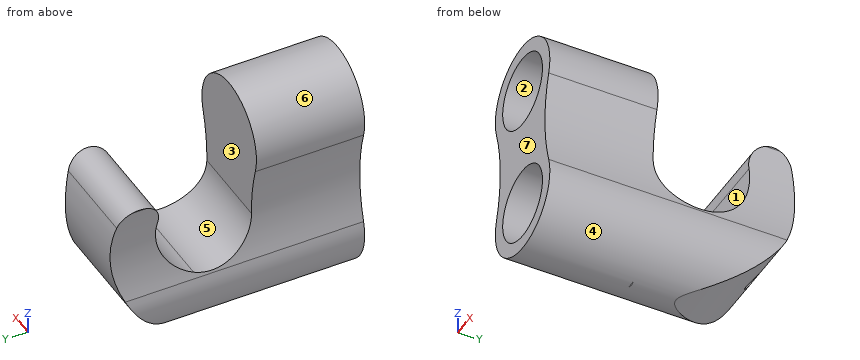
from build123d import *

# Parameters (mm, degrees)
F0_R     = 10.922
F1_DEPTH = 25.4
F2_DEPTH = 6.35
F4_DEPTH = 25.4
F5_DEPTH = 76.2
F6_DEPTH = 25.4
F7_D     = 5.4102
F8_R     = 12.7


with BuildPart() as f1:
    # F0 (on Front) → F1 (new body)
    with BuildSketch(Plane.XZ):
        with BuildLine():
            ThreePointArc((14.3656110791, 14.4652509653), (0, 3.7465), (-14.3656110791, 14.4652509653))
            ThreePointArc((-14.3656110791, 14.4652509653), (-12.2625977878, 0), (-14.3656110791, -14.4652509653))
            ThreePointArc((-14.3656110791, -14.4652509653), (0, -3.7465), (14.3656110791, -14.4652509653))
            ThreePointArc((14.3656110791, -14.4652509653), (12.2625977878, 0), (14.3656110791, 14.4652509653))
        make_face()
        with BuildLine():
            ThreePointArc((14.3656110791, 14.4652509653), (14.8300917669, 16.5764447631), (14.986, 18.7325))
            ThreePointArc((14.986, 18.7325), (-2.1560552369, 33.5625917669), (-14.3656110791, 14.4652509653))
            ThreePointArc((-14.3656110791, 14.4652509653), (0, 3.7465), (14.3656110791, 14.4652509653))
        make_face()
        with Locations((0, 18.7325)):
            Circle(F0_R, mode=Mode.SUBTRACT)
        with BuildLine():
            ThreePointArc((14.3656110791, -14.4652509653), (0, -3.7465), (-14.3656110791, -14.4652509653))
            ThreePointArc((-14.3656110791, -14.4652509653), (-2.1560552369, -33.5625917669), (14.986, -18.7325))
            ThreePointArc((14.986, -18.7325), (14.8300917669, -16.5764447631), (14.3656110791, -14.4652509653))
        make_face()
        with Locations((0, -18.7325)):
            Circle(F0_R, mode=Mode.SUBTRACT)
    extrude(amount=F1_DEPTH)

    # F0 (on Front) → F2 (join)
    with BuildSketch(Plane.XZ):
        with BuildLine():
            ThreePointArc((14.3656110791, 14.4652509653), (14.8300917669, 16.5764447631), (14.986, 18.7325))
            ThreePointArc((14.986, 18.7325), (-2.1560552369, 33.5625917669), (-14.3656110791, 14.4652509653))
            ThreePointArc((-14.3656110791, 14.4652509653), (0, 3.7465), (14.3656110791, 14.4652509653))
        make_face()
        with Locations((0, 18.7325)):
            Circle(F0_R, mode=Mode.SUBTRACT)
        with BuildLine():
            ThreePointArc((14.3656110791, 14.4652509653), (0, 3.7465), (-14.3656110791, 14.4652509653))
            ThreePointArc((-14.3656110791, 14.4652509653), (-12.2625977878, 0), (-14.3656110791, -14.4652509653))
            ThreePointArc((-14.3656110791, -14.4652509653), (0, -3.7465), (14.3656110791, -14.4652509653))
            ThreePointArc((14.3656110791, -14.4652509653), (12.2625977878, 0), (14.3656110791, 14.4652509653))
        make_face()
        with BuildLine():
            ThreePointArc((14.3656110791, -14.4652509653), (0, -3.7465), (-14.3656110791, -14.4652509653))
            ThreePointArc((-14.3656110791, -14.4652509653), (-2.1560552369, -33.5625917669), (14.986, -18.7325))
            ThreePointArc((14.986, -18.7325), (14.8300917669, -16.5764447631), (14.3656110791, -14.4652509653))
        make_face()
        with Locations((0, -18.7325)):
            Circle(F0_R, mode=Mode.SUBTRACT)
        with Locations((0, 18.7325)):
            Circle(F0_R)
        with Locations((0, -18.7325)):
            Circle(F0_R)
    extrude(amount=-F2_DEPTH)

    # F3 (on Right) → F4 (join, symmetric)
    with BuildSketch(Plane.YZ):
        with BuildLine():
            Line((0, 0), (6.35, -33.6685143411))
            ThreePointArc((6.35, -33.6685143411), (38.7816728167, -23.0090487153), (46.444249479, 10.2583907415))
            ThreePointArc((46.444249479, 10.2583907415), (38.5562501556, 14.5507638234), (34.2638770738, 6.6627644999))
            ThreePointArc((34.2638770738, 6.6627644999), (20.4633207868, -13.8005562869), (0, 0))
        make_face()
    extrude(amount=F4_DEPTH, both=True)

    # F0 (on Front) → F5 (intersect)
    with BuildSketch(Plane.XZ):
        with BuildLine():
            ThreePointArc((14.3656110791, 14.4652509653), (14.8300917669, 16.5764447631), (14.986, 18.7325))
            ThreePointArc((14.986, 18.7325), (-2.1560552369, 33.5625917669), (-14.3656110791, 14.4652509653))
            ThreePointArc((-14.3656110791, 14.4652509653), (0, 3.7465), (14.3656110791, 14.4652509653))
        make_face()
        with Locations((0, 18.7325)):
            Circle(F0_R, mode=Mode.SUBTRACT)
        with BuildLine():
            ThreePointArc((14.3656110791, 14.4652509653), (0, 3.7465), (-14.3656110791, 14.4652509653))
            ThreePointArc((-14.3656110791, 14.4652509653), (-12.2625977878, 0), (-14.3656110791, -14.4652509653))
            ThreePointArc((-14.3656110791, -14.4652509653), (0, -3.7465), (14.3656110791, -14.4652509653))
            ThreePointArc((14.3656110791, -14.4652509653), (12.2625977878, 0), (14.3656110791, 14.4652509653))
        make_face()
        with BuildLine():
            ThreePointArc((14.3656110791, -14.4652509653), (0, -3.7465), (-14.3656110791, -14.4652509653))
            ThreePointArc((-14.3656110791, -14.4652509653), (-2.1560552369, -33.5625917669), (14.986, -18.7325))
            ThreePointArc((14.986, -18.7325), (14.8300917669, -16.5764447631), (14.3656110791, -14.4652509653))
        make_face()
        with Locations((0, -18.7325)):
            Circle(F0_R, mode=Mode.SUBTRACT)
        with Locations((0, -18.7325)):
            Circle(F0_R)
        with Locations((0, 18.7325)):
            Circle(F0_R)
    extrude(amount=-F5_DEPTH, mode=Mode.INTERSECT)

    # F0 (on Front) → F6 (join)
    with BuildSketch(Plane.XZ):
        with BuildLine():
            ThreePointArc((14.3656110791, 14.4652509653), (14.8300917669, 16.5764447631), (14.986, 18.7325))
            ThreePointArc((14.986, 18.7325), (-2.1560552369, 33.5625917669), (-14.3656110791, 14.4652509653))
            ThreePointArc((-14.3656110791, 14.4652509653), (0, 3.7465), (14.3656110791, 14.4652509653))
        make_face()
        with Locations((0, 18.7325)):
            Circle(F0_R, mode=Mode.SUBTRACT)
        with BuildLine():
            ThreePointArc((14.3656110791, 14.4652509653), (0, 3.7465), (-14.3656110791, 14.4652509653))
            ThreePointArc((-14.3656110791, 14.4652509653), (-12.2625977878, 0), (-14.3656110791, -14.4652509653))
            ThreePointArc((-14.3656110791, -14.4652509653), (0, -3.7465), (14.3656110791, -14.4652509653))
            ThreePointArc((14.3656110791, -14.4652509653), (12.2625977878, 0), (14.3656110791, 14.4652509653))
        make_face()
        with BuildLine():
            ThreePointArc((14.3656110791, -14.4652509653), (0, -3.7465), (-14.3656110791, -14.4652509653))
            ThreePointArc((-14.3656110791, -14.4652509653), (-2.1560552369, -33.5625917669), (14.986, -18.7325))
            ThreePointArc((14.986, -18.7325), (14.8300917669, -16.5764447631), (14.3656110791, -14.4652509653))
        make_face()
        with Locations((0, -18.7325)):
            Circle(F0_R, mode=Mode.SUBTRACT)
    extrude(amount=F6_DEPTH)

    # F7 (through all)
    with Locations(Plane.XZ):
        with Locations((0, -18.7325)):
            Hole(F7_D / 2)

    # F8
    f8_edges = [f1.edges().sort_by_distance(p)[0] for p in [
        (0, 6.35, -10.392729),
    ]]
    fillet(f8_edges, radius=F8_R)


solid = f1.part
Verification items for the finished model (mm, model axes). Face numbers are marked on the shaded views. A direction names the side the tool comes from. Coordinates: 2 decimals unless noted, no trailing zeros. Loops run counter-clockwise (first coordinate to the right, second up) from the corner with the lowest first, then second, coordinate; pieces in that order, holes last. Notation, with made-up numbers: M -38.75,84 L -26.75,84 A8 cw -26.75,96 Z; hole C 76,-7 d9. An arc over 180 degrees is marked long. One line per item, written item: value.
1. Gauge pin test, flat ends, axial feed: P1, Ø12, axis at x = 4.5, z = -20.5, coming from the -Y side; P2, Ø3, axis at x = -3, y = 18.5, coming from the +Z side; P3, Ø3, axis at x = 9.5, y = -9.5, coming from the +Z side; P4, Ø12, axis at x = 9.5, z = -21, coming from the -Y side. Record the tip position at first contact, or that the pin passes through.
Answers follow:
P1: y = 0
P2: z = -13.55
P3: z = 31.4
P4: y = -25.4
2. Mould release check, pull along Z, two halves, no side actions. Record for the marked faces 5, 6 and 7: pulls with the +Z half, pulls with the -Z half, needs draft (parallel to the pull), parting line crosses it, or undercut.
Answers follow:
face 5: pulls with the +Z half
face 6: undercut
face 7: needs draft
3. Section check C-C on y = 27. Record the cut outline in (x, z).
Answers follow:
outline: M -14.37,-14.47 A14.99 ccw -7.95,-31.44 L 7.95,-31.44 A14.99 ccw 14.37,-14.47 A50.8 cw 13.48,-11.06 L -13.48,-11.06 A50.8 cw Z; hole C 0,-18.73 d5.41
4. Set-up check for the marked faces 1, 2, 3 and 4: record each of +Z, -Z, +X, -X, +Y, -Y from which the full face is reachable in a straight line by a thin tool's end or side.
Answers follow:
face 1: +X, -X
face 2: -Y
face 3: +Z, +X, -X
face 4: +Y, -Y
5. Section check A-A on z = -20. Record the cut outline in (x, y).
Answers follow:
outline: M -14.93,-25.4 L -10.85,-25.4 L -10.85,0 L -2.39,0 L -2.39,41.23 L -14.93,41.23 Z; M 2.39,0 L 10.85,0 L 10.85,-25.4 L 14.93,-25.4 L 14.93,41.23 L 2.39,41.23 Z
6. Section check D-D on z = 20. Record the cut outline in (x, y).
Answers follow:
outline: M -14.93,-25.4 L -10.85,-25.4 L -10.85,0 L 10.85,0 L 10.85,-25.4 L 14.93,-25.4 L 14.93,6.35 L -14.93,6.35 Z
7. Material ranges on line 1 along X through (y, z) = (-12.5, -18.5); line 2 along Z through (x, y) = (0, -9.5); line 3 along Z through (x, y) = (8.5, -2.5), recorded low to high. Write a range as from..to.
Answers follow:
line 1: -14.98..-10.92, 10.92..14.98
line 2: -33.72..-29.65, -7.81..7.81, 29.65..33.72
line 3: -31.07..-25.59, -11.87..11.87, 25.59..31.07
8. Section check B-B on x = 0. Record the cut outline in (y, z), plus the area to 3 significant figures.
Answers follow:
outline: M -25.4,-33.72 L 6.35,-33.72 L 6.35,-33.67 A34.75 ccw 6.61,-33.72 L 19.62,-33.72 A34.75 ccw 40.13,-21.44 L 0,-21.44 L 0,-29.65 L -25.4,-29.65 Z; M -25.4,-7.81 L 0,-7.81 L 0,-16.03 L 43.73,-16.03 A34.75 ccw 46.44,10.26 A6.35 ccw 34.26,6.66 A17.45 cw 24.18,-12.64 A12.7 cw 6.35,-1.02 L 6.35,33.72 L -25.4,33.72 L -25.4,29.65 L 0,29.65 L 0,7.81 L -25.4,7.81 Z
area: 1,840 mm^2
